Work out the finished part from the listing and answer in its coordinate system (mm). A direction names the side the tool comes from. Coordinates: 2 decimals unless noted, no trailing zeros. Loops run counter-clockwise (first coordinate to the right, second up) from the corner with the lowest first, then second, coordinate; pieces in that order, holes last. Notation, with made-up numbers: (50, 0.25) -> (103, 0.25) arc R20 ccw to (103, 5.25) -> close; hole circle Ø9 at (0, 26.5). An arc over 180 degrees is marked (long way). One line per question, with ' | ' between items.
```python
from build123d import *

# Parameters (mm, degrees)
SKETCH1_W               = 105
SKETCH1_H               = 85
SKETCH1_R               = 4
BOSS_EXTRUDE1_DEPTH     = 10
FILLET1_R               = 7
FILLET2_R               = 7
SKETCH17_R              = 18
SKETCH17_R_2            = 17
BOSS_EXTRUDE2_DEPTH     = 700
RIB2_REACH              = 715.206
SKETCH18_WALL_W         = 1447.913707502
SKETCH18_WALL_H         = 4
CIRPATTERN1_COUNT       = 4
CUT_EXTRUDE1_REACH      = 716.504
CUT_EXTRUDE1_END_RADIUS = 17
SKETCH19_R              = 4.1


with BuildPart() as part:
    # Sketch1 → Boss-Extrude1 (new body)
    with BuildSketch(Plane(origin=(0, 0, 0), x_dir=(1, 0, 0), z_dir=(0, 1, 0))):
        Rectangle(SKETCH1_W, SKETCH1_H)
        with Locations(Location((-40, -30, 0), (0, 0, 270))):
            Circle(SKETCH1_R, mode=Mode.SUBTRACT)
        with Locations(Location((40, 30, 0), (0, 0, 270))):
            Circle(SKETCH1_R, mode=Mode.SUBTRACT)
        with Locations(Location((40, -30, 0), (0, 0, 270))):
            Circle(SKETCH1_R, mode=Mode.SUBTRACT)
        with Locations(Location((-40, 30, 0), (0, 0, 270))):
            Circle(SKETCH1_R, mode=Mode.SUBTRACT)
    extrude(amount=BOSS_EXTRUDE1_DEPTH)

    # Fillet1
    fillet1_edges = [part.edges().sort_by_distance(p)[0] for p in [
        (52.5, 10, 0),
        (-52.5, 10, 0),
        (52.5, 5, 42.5),
        (-52.5, 5, 42.5),
    ]]
    fillet(fillet1_edges, radius=FILLET1_R)

    # Fillet2
    # the kernel refuses this fillet: 7 mm, written as the material it takes off along each edge
    with BuildSketch(Plane(origin=(45.5, 3, 35.5), x_dir=(0, 1, 0), z_dir=(0, 0, 1))) as fillet2_piece_1_section:
        Polygon((0, 0), (FILLET2_R, 0), (FILLET2_R, -FILLET2_R), (0, -FILLET2_R), align=None)
    fillet2_piece_1 = extrude(amount=FILLET2_R, mode=Mode.PRIVATE)
    fillet2_piece_1 = fillet2_piece_1 - Plane(origin=(45.5, 3, 35.5), x_dir=(-0.7071067811865475, -0.7071067811865475, 0), z_dir=(0, 0, 1)) * Sphere(FILLET2_R, mode=Mode.PRIVATE)
    add(fillet2_piece_1, mode=Mode.SUBTRACT)
    with BuildSketch(Plane(origin=(-45.5, 3, 35.5), x_dir=(0, 1, 0), z_dir=(0, 0, 1))) as fillet2_piece_2_section:
        Polygon((0, 0), (FILLET2_R, 0), (FILLET2_R, FILLET2_R), (0, FILLET2_R), align=None)
    fillet2_piece_2 = extrude(amount=FILLET2_R, mode=Mode.PRIVATE)
    fillet2_piece_2 = fillet2_piece_2 - Plane(origin=(-45.5, 3, 35.5), x_dir=(0.7071067811865475, -0.7071067811865475, 0), z_dir=(0, 0, 1)) * Sphere(FILLET2_R, mode=Mode.PRIVATE)
    add(fillet2_piece_2, mode=Mode.SUBTRACT)
    with BuildSketch(Plane(origin=(45.5, 10, 42.5), x_dir=(0, -1, 0), z_dir=(-1, 0, 0))) as fillet2_piece_3:
        with BuildLine():
            CenterArc((FILLET2_R, -FILLET2_R), FILLET2_R, 90, 90)
            Line((0, -FILLET2_R), (0, 0))
            Line((0, 0), (FILLET2_R, 0))
        make_face()
    extrude(amount=91, mode=Mode.SUBTRACT)
    with BuildSketch(Plane(origin=(-45.5, 10, -42.5), x_dir=(0, 0, 1), z_dir=(1, 0, 0))) as fillet2_piece_4:
        with BuildLine():
            CenterArc((FILLET2_R, FILLET2_R), FILLET2_R, 180, 90)
            Line((0, FILLET2_R), (0, 0))
            Line((0, 0), (FILLET2_R, 0))
        make_face()
    extrude(amount=91, mode=Mode.SUBTRACT)
    with BuildSketch(Plane(origin=(-52.5, -17.5, -42.5), x_dir=(0, 0, 1), z_dir=(0, 1, 0))) as fillet2_piece_5:
        with BuildLine():
            CenterArc((FILLET2_R, FILLET2_R), FILLET2_R, 180, 90)
            Line((0, FILLET2_R), (0, 0))
            Line((0, 0), (FILLET2_R, 0))
        make_face()
    extrude(amount=20.5, mode=Mode.SUBTRACT)
    with BuildSketch(Plane(origin=(52.5, -17.5, -42.5), x_dir=(0, 0, 1), z_dir=(0, 1, 0))) as fillet2_piece_6:
        with BuildLine():
            CenterArc((FILLET2_R, -FILLET2_R), FILLET2_R, 90, 90)
            Line((0, -FILLET2_R), (0, 0))
            Line((0, 0), (FILLET2_R, 0))
        make_face()
    extrude(amount=20.5, mode=Mode.SUBTRACT)
    with BuildSketch(Plane(origin=(-45.5, 3, -42.5), x_dir=(-1, 0, 0), z_dir=(0, -1, 0))) as fillet2_piece_7:
        with BuildLine():
            CenterArc((7 - FILLET2_R, -FILLET2_R), FILLET2_R, 0, 90)
            Line((7, -FILLET2_R), (7, 0))
            Line((7, 0), (7 - FILLET2_R, 0))
        make_face()
    revolve(axis=Axis((-45.5, 3, -42.5), (0, 0, -1)), revolution_arc=90, mode=Mode.SUBTRACT)
    with BuildSketch(Plane(origin=(45.5, 3, -42.5), x_dir=(1, 0, 0), z_dir=(0, -1, 0))) as fillet2_piece_8:
        with BuildLine():
            CenterArc((7 - FILLET2_R, FILLET2_R), FILLET2_R, 270, 90)
            Line((7, FILLET2_R), (7, 0))
            Line((7, 0), (7 - FILLET2_R, 0))
        make_face()
    revolve(axis=Axis((45.5, 3, -42.5), (0, 0, 1)), revolution_arc=90, mode=Mode.SUBTRACT)

    # Sketch17 → Boss-Extrude2 (add)
    with BuildSketch(Plane(origin=(0, 10, 0), x_dir=(1, 0, 0), z_dir=(0, 1, 0))):
        with Locations(Location((0, 0, 0), (0, 0, 270))):
            Circle(SKETCH17_R)
        with Locations(Location((0, 0, 0), (0, 0, 270))):
            Circle(SKETCH17_R_2, mode=Mode.SUBTRACT)
    extrude(amount=BOSS_EXTRUDE2_DEPTH)

    # Sketch18 wall → Rib2 (add, up to next)
    with BuildSketch(Plane(origin=(-24.522935069, 16.901577145, 0), x_dir=(-0.707106781187, -0.707106781187, 0), z_dir=(0.707106781187, -0.707106781187, 0)), mode=Mode.PRIVATE) as rib2_sk1:
        Rectangle(SKETCH18_WALL_W, SKETCH18_WALL_H)
    rib2_tool1 = extrude(rib2_sk1.sketch, amount=RIB2_REACH, mode=Mode.PRIVATE) - part.part
    rib2 = rib2_tool1.solids().sort_by_distance((-24.522935069, 16.901577145, 0))[0]
    add(rib2)

    # CirPattern1: Rib2 ×4 about axis
    cirpattern1_axis = Axis((0, 0, 0), (0, 1, 0))
    for i in range(1, CIRPATTERN1_COUNT):
        add(rib2.rotate(cirpattern1_axis, i * 360 / CIRPATTERN1_COUNT))

    # Cut-Extrude1: up to this cylinder (the profile starts outside it)
    cut_extrude1_end = Plane(origin=(0, 660, 0), z_dir=(0, -1, 0)) * Cylinder(CUT_EXTRUDE1_END_RADIUS, 1468.008, mode=Mode.PRIVATE)
    # Sketch19 → Cut-Extrude1 (cut, up to the surface)
    with BuildSketch(Plane.XY.offset(18), mode=Mode.PRIVATE) as cut_extrude1_sk1:
        with Locations((0, 660)):
            Circle(SKETCH19_R)
    cut_extrude1_tool1 = extrude(cut_extrude1_sk1.sketch, amount=-CUT_EXTRUDE1_REACH, mode=Mode.PRIVATE) - cut_extrude1_end
    add(cut_extrude1_tool1.solids().sort_by_distance((0, 660, 18))[0], mode=Mode.SUBTRACT)


solid = part.part
```
1) Find section B-B (x = 25.5). Write down the section's boundary in (y, z).
Check values:
outline: (0, -42.5) -> (3, -42.5) arc R7 ccw to (10, -35.5) -> (10, -2) -> (15.92, -2) -> (15.92, 2) -> (10, 2) -> (10, 35.5) arc R7 ccw to (3, 42.5) -> (0, 42.5) -> close
2) Find section C-C (z = -8). Write down the section's boundary in (x, y).
Check values:
outline: (-52.5, 0) -> (52.5, 0) -> (52.5, 3) arc R7 ccw to (45.5, 10) -> (16.12, 10) -> (16.12, 710) -> (15, 710) -> (15, 10) -> (-15, 10) -> (-15, 710) -> (-16.12, 710) -> (-16.12, 10) -> (-45.5, 10) arc R7 ccw to (-52.5, 3) -> close
3) Flat-ended cylindrical pins translate along their axes: pin 1 (6.5 mm diameter, centred on x = 40, z = 30, fed in from +Y); pin 2 (12 mm diameter, centred on x = 12.5, y = 634.5, fed in from +Z); pin 3 (6 mm diameter, centred on x = 13.5, y = 585, fed in from +Z); pin 4 (6.5 mm diameter, centred on x = 0, y = 660, fed in from -Z). Find the tip coordinate at first contact, or state that the pin passes through.
Check values:
pin 1: passes through | pin 2: stops at z = 16.79 | pin 3: stops at z = 14.62 | pin 4: stops at z = -18
4) The mould has two halves that part along X. Classify faces 4 (the face through (5.106, 355.1, 16.215)), 5 (the face through (-24.562, 16.863, -0.028)), 6 (the face through (-22, 14, -2)), 7 (the face through (0, 10, 0)): released by +X, released by -X, zero draft, split by the parting line, or undercut.
Check values:
face 4: undercut | face 5: released by -X | face 6: zero draft | face 7: undercut
5) Find section A-A (y = 488). Write down the section's boundary in (x, z).
Check values:
outline: circle Ø36 at (0, 0); hole circle Ø34 at (0, 0)
6) For faces 1 (the face through (2, 14, 22)), 2 (the face through (-22, 14, 2)), 3 (the face through (2, 14, -22)), determine the directions among +Z, -Z, +X, -X, +Y, -Y from which every point of the face is accessible in a straight line to the end or side of a thin tool.
Check values:
face 1: +Z, +X, +Y | face 2: +Z, -X, +Y | face 3: -Z, +X, +Y
7) Find the intervals of material crossed by line 1 along X through (y, z) = (3.75, 30); line 2 along Y through (x, z) = (0, 17.15); line 3 along X through (y, z) = (7, 30), in increasing order.
Check values:
line 1: x = -52.46 to -44, -36 to 36, 44 to 52.46 | line 2: y = 0 to 655.9, 664.1 to 710 | line 3: x = -51.24 to -44, -36 to 36, 44 to 51.24
